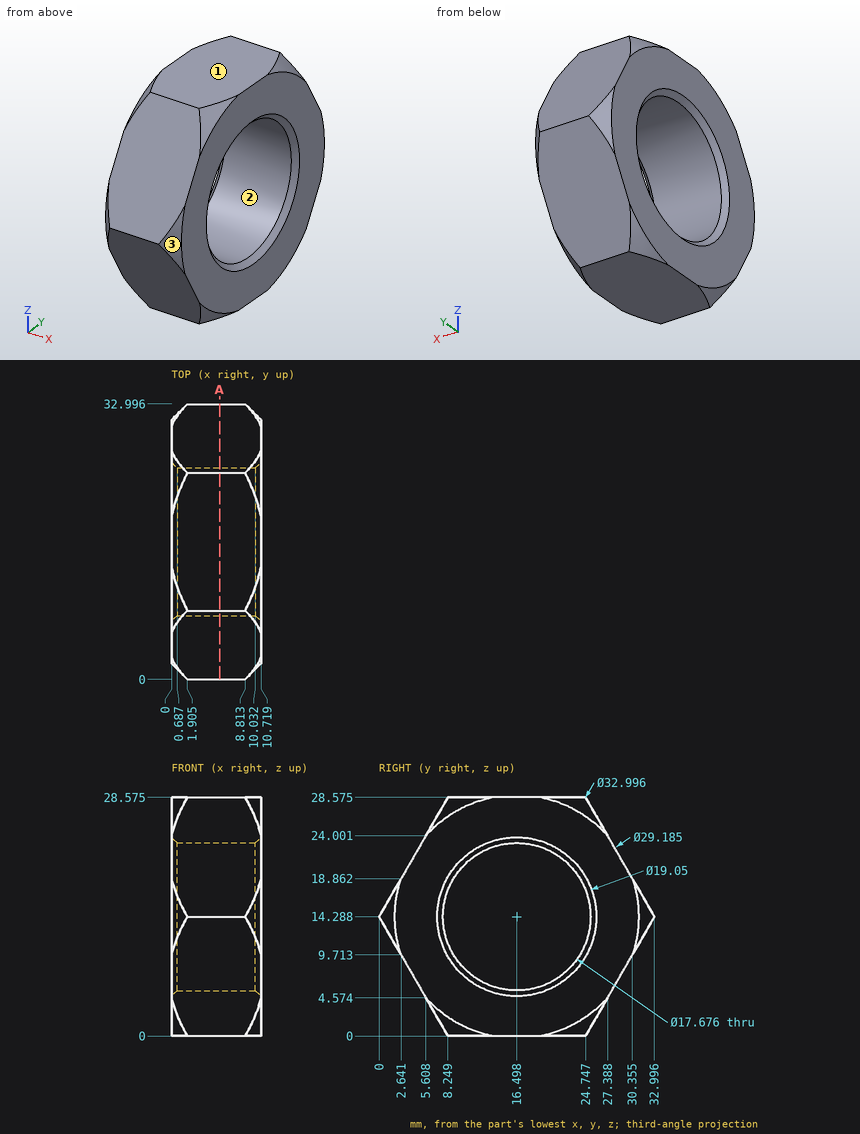
Can you work these out from the drawing? Everything is in mm from the part's minimum corner. Round coordinates to 2 decimals unless told otherwise and drop trailing zeros. Loops run counter-clockwise (first coordinate to the right, second up) from the corner with the lowest first, then second, coordinate; pieces in that order, holes last. Notation, with made-up numbers: (74.5, -31) -> (129.5, -31) arc R20 ccw to (129.5, -23) -> close; hole circle Ø4 at (2.25, 68.25). An arc over 180 degrees is marked (long way). Put each result on its own line as item: value.
Q1. Thinking about a two-plate mould opening in Y: for the marked faces 1, 2 and 3, which applies, pulls with the +Y half, pulls with the -Y half, needs draft (parallel to the pull), parting line crosses it, or undercut?
Checks:
face 1: needs draft
face 2: undercut
face 3: pulls with the -Y half
Q2. For pin 1 Ø1 at (x, z) = (9, 10.5) entering from +Y; pin 2 Ø2 at (x, z) = (3.5, 21) entering from +Y; pin 3 Ø1 at (x, z) = (4.5, 24.5) entering from -Y, each with a flat end and sliding along its axis, tell me the tip position at first contact or that it passes through.
Checks:
pin 1: y = 31.1
pin 2: y = 29.7
pin 3: y = 5.61
Q3. Please list where these lines run through material, in increasing order: line 1 (Z direction, x = 9, y = 18) (1 decimal); line 2 (Z direction, x = 6.75, y = 22) (1 decimal); line 3 (Y direction, x = 1.25, z = 18.25). Write a range as from..to.
Checks:
line 1: 0..5.6, 23..28.6
line 2: 0..7.4, 21.2..28.6
line 3: 2.29..8.6, 24.4..30.71
Q4. I want a section at A-A on x = 5.75. Write out the boundary of the cut face in (y, z) (1 decimal), and give its area (3 significant figures).
Checks:
outline: (0, 14.3) -> (8.2, 0) -> (24.7, 0) -> (33, 14.3) -> (24.7, 28.6) -> (8.2, 28.6) -> close; hole circle Ø17.7 at (16.5, 14.3)
area: 462 mm2
